The model under review builds one solid part; all positions refer to its coordinate system, in mm. Face numbers are marked on the shaded views. Give positions to 0.01 mm unless a question says otherwise; leave off trailing zeros. Write each loop counter-clockwise with the first axis right and the second up, starting at its lowest first coordinate (ties: lowest second). Pieces come first, ordered by that corner, then holes. Notation, with made-up numbers: M 87,6.25 L 116,6.25 A20 cw 116,38.25 Z; hole C 7.25,-30 d7. An arc over 180 degrees is marked long. Write item = value, one per line. Start each with the question number.
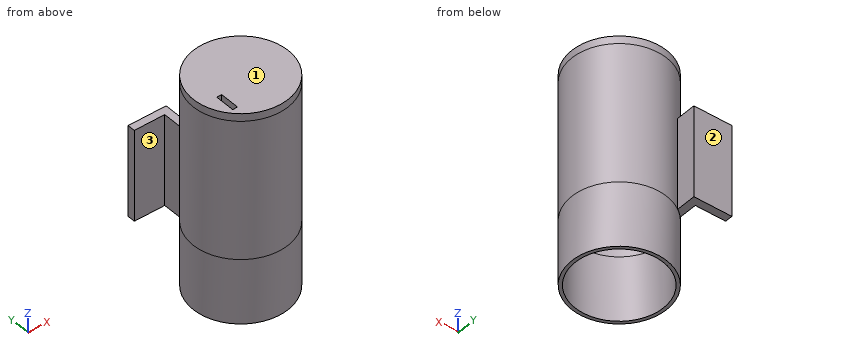
```python
from build123d import *

# Parameters (mm, degrees)
SKETCH1_W                = 12.7
SKETCH1_H                = 3.175
SKETCH1_W_2              = 3.175
SKETCH1_H_2              = 11
BOSS_EXTRUDE1_DEPTH      = 38.1
SKETCH2_R                = 19.784587186
SKETCH2_R_2              = 18.4
BOSS_EXTRUDE2_DEPTH      = 27
BOSS_EXTRUDE2_DEPTH_BACK = 58
SKETCH3_R                = 19.784587186
BOSS_EXTRUDE3_DEPTH      = 3.175
SKETCH4_W                = 2.053355329
SKETCH4_H                = 8.144976138
CUT_EXTRUDE1_DEPTH       = 3.175


with BuildPart() as part:
    # Sketch1 → Boss-Extrude1 (new body)
    with BuildSketch(Plane.XY):
        with Locations((-16.162006615, 10.28820212)):
            Rectangle(SKETCH1_W, SKETCH1_H)
        with Locations((-8.224506615, 6.37570212)):
            Rectangle(SKETCH1_W_2, SKETCH1_H_2)
    extrude(amount=BOSS_EXTRUDE1_DEPTH)

    # Sketch2 → Boss-Extrude2 (add, two sides)
    with BuildSketch(Plane(origin=(0, 0, 0), x_dir=(-1, 0, 0), z_dir=(0, 0, -1))) as boss_extrude2_sk:
        with Locations((-4.329778131, -12.861954284)):
            Circle(SKETCH2_R)
        with Locations((-4.329778131, -12.861954284)):
            Circle(SKETCH2_R_2, mode=Mode.SUBTRACT)
    extrude(amount=BOSS_EXTRUDE2_DEPTH)
    extrude(boss_extrude2_sk.sketch, amount=-BOSS_EXTRUDE2_DEPTH_BACK)

    # Sketch3 → Boss-Extrude3 (add)
    with BuildSketch(Plane.XY.offset(58)):
        with Locations((4.329778131, -12.861954284)):
            Circle(SKETCH3_R)
    extrude(amount=BOSS_EXTRUDE3_DEPTH)

    # Sketch4 → Cut-Extrude1 (cut)
    with BuildSketch(Plane.XY.offset(61.175)):
        with Locations((-7.822913032, -20.823309264)):
            Rectangle(SKETCH4_W, SKETCH4_H)
    extrude(amount=-CUT_EXTRUDE1_DEPTH, mode=Mode.SUBTRACT)


solid = part.part
```
Item 1: The part is to be moulded in two halves that separate along Y. For the marked faces 1, 2 and 3, say which applies: released by +Y, released by -Y, zero draft, split by the parting line, or undercut.
Item 2: We need section B-B, the plane y = -19. Write out the cut boundary in (x, z) (3 decimals).
Item 3: We need section C-C, the plane x = -13. Write out the cut boundary in (y, z) (3 decimals).
Item 4: We need section A-A, the plane z = 20.5. Write out the cut boundary in (x, y), and give its area (3 significant figures).
Item 5: We need section D-D, the plane x = -0.5. Write out the cut boundary in (y, z) (3 decimals).
Item 6: Clearance check with flat-ended pins moving along their axes: P1, Ø3.5, axis at y = -19, z = 59.5, coming from the +X side; P2, Ø0.6, axis at x = -7.5, z = 59, coming from the -Y side; P3, Ø12, axis at x = -15.5, y = 5.5, coming from the -Z side. State where each tip first meets the part, or that it passes through.
Item 7: To check wall thickness, follow probe 1 along Z at (x, y) = (-2, -29.5) (3 decimals); probe 2 along X at (y, z) = (-4, -22); probe 3 along Y at (x, z) = (17.5, 12). State the ranges of each line that lie inside material, in increasing order. Write a range as [from, to].
Worked out:
q1.face_1 = zero draft
q1.face_2 = released by +Y
q1.face_3 = undercut
q2.outline = M -14.479,-27 L -13.016,-27 L -13.016,58 L -8.85,58 L -8.85,61.175 L -14.479,61.175 Z; M -6.796,58 L 21.676,58 L 21.676,-27 L 23.138,-27 L 23.138,61.175 L -6.796,61.175 Z
q3.outline = M -22.407,-27 L -19.046,-27 L -19.046,58 L -6.678,58 L -6.678,-27 L -3.317,-27 L -3.317,61.175 L -22.407,61.175 Z; M 8.701,0 L 11.876,0 L 11.876,38.1 L 8.701,38.1 Z
q4.outline = M -22.51,8.7 L -9.81,8.7 L -9.81,0.97 A19.78 ccw long -6.64,3.6 L -6.64,11.88 L -22.51,11.88 Z; hole M -7.91,0.88 A18.4 ccw long -6.64,1.91 L -6.64,0.88 Z
q4.area = 237 mm²
q5.outline = M -32.048,-27 L -30.617,-27 L -30.617,58 L 4.893,58 L 4.893,-27 L 6.324,-27 L 6.324,61.175 L -32.048,61.175 Z
q6.P1 = 23.62
q6.P2 = -28.94
q6.P3 = 0
q7.probe_1 = [58, 61.175]
q7.probe_2 = [-13.36, -11.8], [20.46, 22.02]
q7.probe_3 = [-27.63, -25.71], [-0.01, 1.9]
